Check sheet for the modelled part. Datum: model origin and axes. Units: mm. Face numbers are marked on the shaded views. Round coordinates to 2 decimals unless told otherwise and drop trailing zeros. Order: outer loops, then holes, each group sorted by start corner. A loop starts at its lowest first (then second) coordinate and runs counter-clockwise, first axis right, second up.
(1) Sectioned sample at B-B, the plane y = 22. Enter the section's corners in (x, z).
(2) Mould release check, pull along X, two halves, no side actions. Record for the marked faces 1, 2 and 3: released by +X, released by -X, zero draft, split by the parting line, or undercut.
(3) Sectioned sample at C-C, the plane z = -33. Enter the section's corners in (x, y), and give its area (3 significant figures).
(4) Thickness scan on probe 1 along Z at (x, y) = (-21.5, 35); probe 2 along Y at (x, z) = (-22.5, -17); probe 3 along Y at (x, z) = (36.5, -40). Record the ranges inside material, lowest first.
(5) Depth check by flat-ended pin: pin 1 (6 mm diameter, centred on y = 24.5, z = -20, fed in from +X); pin 2 (5 mm diameter, centred on x = -7.5, z = -12.5, fed in from +Y); pin 3 (12 mm diameter, centred on x = -21.5, y = 20, fed in from -Z); pin 4 (6 mm diameter, centred on x = -6, z = -37, fed in from +Y). Enter the tip coordinate at first touch or a pass-through.
(6) Sectioned sample at A-A, the plane x = -17. Enter the section's corners in (y, z), and give its area (3 significant figures).
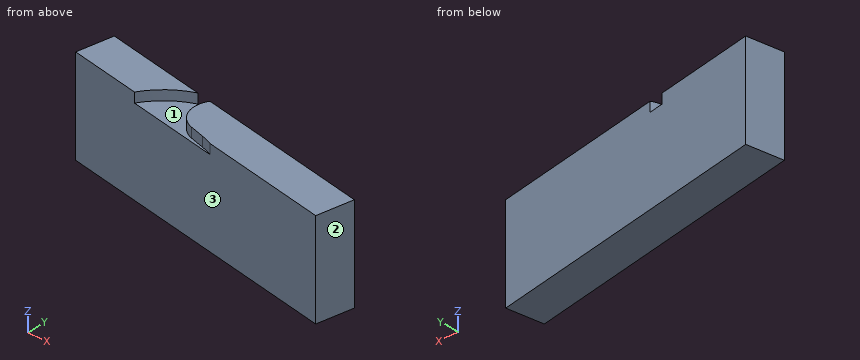
```python
from build123d import *

# Parameters (mm, degrees)
BOSS_EXTRUDE1_DEPTH        = 3.048
BOSS_EXTRUDE2_DEPTH        = 2.032
BOSS_EXTRUDE2_DEPTH_BACK   = 47.752
BOSS_EXTRUDE2_2_DEPTH      = 2.032
BOSS_EXTRUDE2_2_DEPTH_BACK = 47.752


with BuildPart() as part:
    # Sketch1 → Boss-Extrude1 (new, symmetric)
    with BuildSketch(Plane.XY):
        with BuildLine():
            ThreePointArc((0, 27.535484012), (-9.412998127, 39.802742006), (0, 52.07))
            Line((0, 52.07), (-11.040532194, 49.111698314))
            ThreePointArc((-11.040532194, 49.111698314), (-39.066320922, 14.192289272), (-14.190605813, -23.03684931))
            Line((-14.190605813, -23.03684931), (0, -28.201807432))
            ThreePointArc((0, -28.201807432), (8.35634418, -40.135903716), (0, -52.07))
            Line((0, -52.07), (10.740686656, -48.160709762))
            ThreePointArc((10.740686656, -48.160709762), (36.144496882, -10.141220984), (7.52373904, 25.519504212))
            Line((7.52373904, 25.519504212), (0, 27.535484012))
        make_face()
        with BuildLine():
            Line((-12.7, 7.332348419), (-1.374815329, 13.870946837))
            ThreePointArc((-1.374815329, 13.870946837), (-0.410875234, 16.198104087), (1.5875, 14.664696837))
            ThreePointArc((1.5875, 14.664696837), (1.533407249, 14.253821603), (1.374815329, 13.870946837))
            Line((1.374815329, 13.870946837), (12.7, 7.332348419))
            Line((12.7, 7.332348419), (12.7, -7.332348419))
            Line((12.7, -7.332348419), (0, -14.664696837))
            Line((0, -14.664696837), (-12.7, -7.332348419))
            Line((-12.7, -7.332348419), (-12.7, 7.332348419))
        make_face(mode=Mode.SUBTRACT)
    extrude(amount=BOSS_EXTRUDE1_DEPTH, both=True)


with BuildPart() as body_2:
    # Sketch2 → Boss-Extrude2 (new, two sides: drawn at the far end of the back side and taken through both)
    with BuildSketch(Plane.XY.offset(-BOSS_EXTRUDE2_DEPTH_BACK)):
        Polygon((-70.631687067, 38.246108065), (79.453014492, 11.782125788), (82.761012277, 30.542713483), (-67.323689282, 57.00669576), align=None)
    extrude(amount=BOSS_EXTRUDE2_DEPTH + BOSS_EXTRUDE2_DEPTH_BACK)


with BuildPart() as body_3:
    # Sketch2 → Boss-Extrude2 2 (new, two sides: drawn at the far end of the back side and taken through both)
    with BuildSketch(Plane.XY.offset(-BOSS_EXTRUDE2_2_DEPTH_BACK)):
        Polygon((-79.453014492, -11.782125788), (70.631687067, -38.246108065), (67.323689282, -57.00669576), (-82.761012277, -30.542713483), align=None)
    extrude(amount=BOSS_EXTRUDE2_2_DEPTH + BOSS_EXTRUDE2_2_DEPTH_BACK)


with BuildPart() as body_2_1:
    add(body_2.part)

    # Intersect1: read off the stored shape, not the designer's step
    # Intersect1: cut body 3, part
    add(body_3.part, mode=Mode.SUBTRACT)
    add(part.part, mode=Mode.SUBTRACT)


solid = body_2_1.part
```
Derived:
1. outline: (21.5, -47.75) - (81.25, -47.75) - (81.25, 2.03) - (21.5, 2.03) - close
2. face 1: undercut
2. face 2: released by +X
2. face 3: released by -X
3. outline: (-70.63, 38.25) - (79.45, 11.78) - (82.76, 30.54) - (-67.32, 57.01) - close
3. area: 2,900 mm2
4. probe 1: z = -47.75 to -3.05
4. probe 2: y = 29.76 to 49.1
4. probe 3: y = 19.36 to 38.7
5. pin 1: stops at x = 82.22
5. pin 2: stops at y = 46.9
5. pin 3: passes through
5. pin 4: stops at y = 46.72
6. outline: (28.79, -47.75) - (48.13, -47.75) - (48.13, 2.03) - (46.97, 2.03) - (46.97, -3.05) - (28.79, -3.05) - close
6. area: 871 mm2
